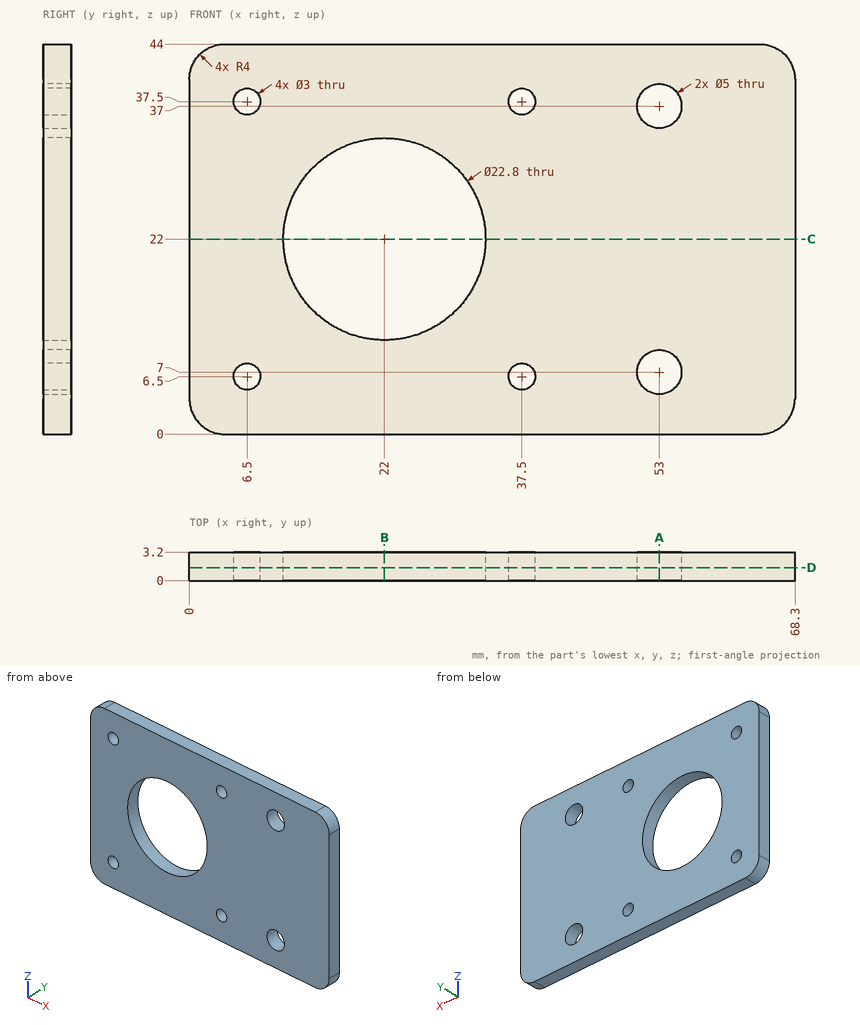
Here's the drawing with two shaded views (mm, measured from the low corner). I have some questions. Coordinates: 2 decimals unless noted, no trailing zeros. Order: outer loops, then holes, each group sorted by start corner. A loop starts at its lowest first (then second) coordinate and runs counter-clockwise, first axis right, second up.
Q1. Suppose I cut it at B-B on x = 22. Please give me the cut outline in (y, z).
Q2. Suppose I cut it at D-D on y = 1.45. Please give me the cut outline in (x, z), and give its area (3 significant figures).
Q3. Suppose I cut it at A-A on x = 53. Please give me the cut outline in (y, z).
Q4. Please list where these lines run through material, in increasing order: L1, parallel to X at y = 1.7, z = 22; L2, parallel to X at y = 1.1, z = 6.5; L3, parallel to Z at x = 53.5, y = 2.4.
Q5. Will this pin go through, and if not, where does the flat tip stop? pin 1 (4 mm diameter, centred on x = 37.5, z = 6.5, fed in from -Y).
Q6. Suppose I cut it at C-C on z = 22. Please give me the cut outline in (x, y), and give its area (3 significant figures).
Answer:
1. outline: (0, 0) - (3.2, 0) - (3.2, 10.6) - (0, 10.6) - close; (0, 33.4) - (3.2, 33.4) - (3.2, 44) - (0, 44) - close
2. outline: (0, 4) arc R4 ccw to (4, 0) - (64.3, 0) arc R4 ccw to (68.3, 4) - (68.3, 40) arc R4 ccw to (64.3, 44) - (4, 44) arc R4 ccw to (0, 40) - close; hole circle Ø3 at (6.5, 6.5); hole circle Ø3 at (6.5, 37.5); hole circle Ø22.8 at (22, 22); hole circle Ø3 at (37.5, 6.5); hole circle Ø3 at (37.5, 37.5); hole circle Ø5 at (53, 7); hole circle Ø5 at (53, 37)
2. area: 2,520 mm2
3. outline: (0, 0) - (3.2, 0) - (3.2, 4.5) - (0, 4.5) - close; (0, 9.5) - (3.2, 9.5) - (3.2, 34.5) - (0, 34.5) - close; (0, 39.5) - (3.2, 39.5) - (3.2, 44) - (0, 44) - close
4. L1: x = 0 to 10.6, 33.4 to 68.3
4. L2: x = 0 to 5, 8 to 36, 39 to 50.55, 55.45 to 68.3
4. L3: z = 0 to 4.55, 9.45 to 34.55, 39.45 to 44
5. pin 1: stops at y = 0
6. outline: (0, 0) - (10.6, 0) - (10.6, 3.2) - (0, 3.2) - close; (33.4, 0) - (68.3, 0) - (68.3, 3.2) - (33.4, 3.2) - close
6. area: 146 mm2
